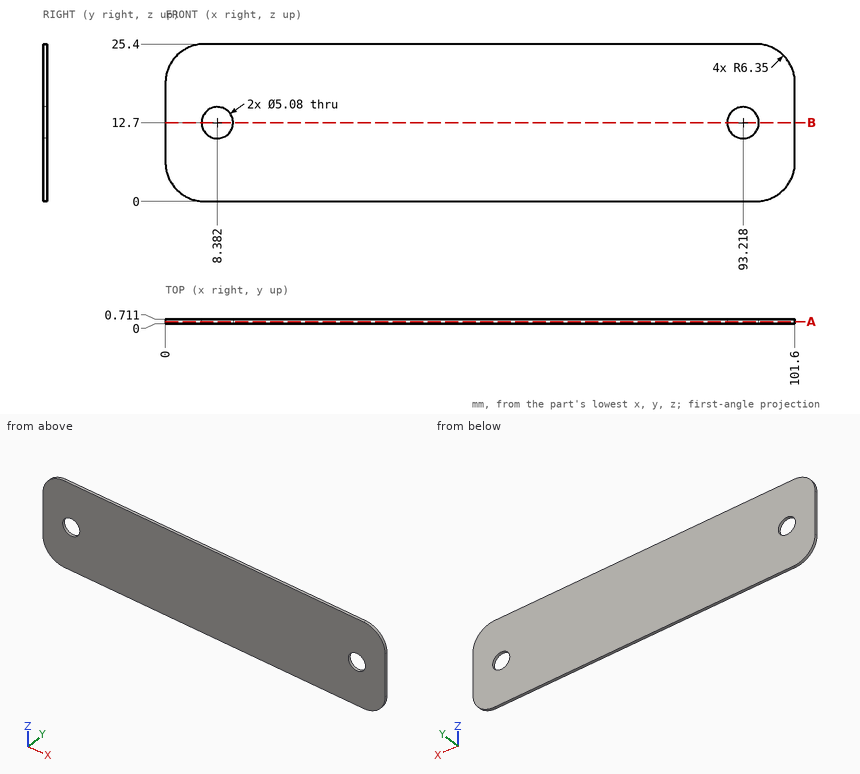
Part print with two shaded views. Sizes in mm from the minimum x, y, z corner. Coordinates: 2 decimals unless noted, no trailing zeros. Write each loop counter-clockwise with the first axis right and the second up, starting at its lowest first coordinate (ties: lowest second). Pieces come first, ordered by that corner, then holes.
(1) Cut at A-A on y = 0.35. List the corners of the cut face in (x, z), and give its area (3 significant figures).
(2) Drill centre lines: line 1 (Z direction, x = 93, y = 0.5); line 2 (Z direction, x = 10.5, y = 0.6); line 3 (Z direction, x = 97, y = 0.65). Where is each one in solid material? Low to high.
(3) Cut at B-B on z = 12.7. List the corners of the cut face in (x, y).
Working result:
1. outline: (0, 6.35) arc R6.35 ccw to (6.35, 0) - (95.25, 0) arc R6.35 ccw to (101.6, 6.35) - (101.6, 19.05) arc R6.35 ccw to (95.25, 25.4) - (6.35, 25.4) arc R6.35 ccw to (0, 19.05) - close; hole circle Ø5.08 at (8.38, 12.7); hole circle Ø5.08 at (93.22, 12.7)
1. area: 2,510 mm2
2. line 1: z = 0 to 10.17, 15.23 to 25.4
2. line 2: z = 0 to 11.3, 14.1 to 25.4
2. line 3: z = 0.25 to 25.15
3. outline: (0, 0) - (5.84, 0) - (5.84, 0.71) - (0, 0.71) - close; (10.92, 0) - (90.68, 0) - (90.68, 0.71) - (10.92, 0.71) - close; (95.76, 0) - (101.6, 0) - (101.6, 0.71) - (95.76, 0.71) - close
